Part model, mm, in its own coordinate system. A direction names the side the tool comes from. Coordinates: 2 decimals unless noted, no trailing zeros. Loops run counter-clockwise (first coordinate to the right, second up) from the corner with the lowest first, then second, coordinate; pieces in that order, holes last. Notation, with made-up numbers: M 55.25,64 L 62.25,64 A23 cw 62.25,84 Z; hole C -8,48 d10. An arc over 180 degrees is marked long. Use a Markdown table: item, result. Add a question column.
1) Band-saw the part on B-B (z = 39.65). List the corners of the cut face in (x, y), plus the area to 3 significant figures.
2) Tool access for faces 5 (the cylindrical face through (77.914, 10.793, 41.254)), 6 (the cylindrical face through (79.71, 37.57, 40.27)): list every direction of +Z, -Z, +X, -X, +Y, -Y with a clear straight run to the whole face (end or side of a thin tool).
3) Band-saw the part on C-C (x = 78.5). List the corners of the cut face in (y, z).
4) Pull direction X, two halves, no side cores. Call faces 1 (the cylindrical face through (80.873, 10.738, 40.268)), 2 (the cylindrical face through (79.419, 45.014, 40.014)), 3 (the flat face through (81, 10, 41.5)), 4 (the cylindrical face through (79.77, 36.52, 40.01)): released by +X, released by -X, zero draft, split by the parting line, or undercut.
5) Pin check, flat tips, straight feed: pin 1 Ø10 at (x, y) = (88.5, 14.5) entering from +Z; pin 2 Ø8 at (x, y) = (79.98, 30.02) entering from +Z. Stop position of each tip, or through.
6) Band-saw the part on A-A (y = 32). List the corners of the cut face in (x, z).
7) Band-saw the part on D-D (y = 37). List the corners of the cut face in (x, z), plus the area to 3 significant figures.
8) Wall check: probe 1 along X at (y, z) = (13, 39.1); probe 2 along Z at (x, y) = (92.5, 23.5); probe 3 along Y at (x, z) = (80.75, 39.5). Give the ranges that are in metal, low to high. Write a range as from..to.
from build123d import *

# Parameters (mm, degrees)
CYLINDER003001001005001001_R     = 3.5
CYLINDER003001001005001001_DEPTH = 2
CYLINDER003001001004002_R        = 1
CYLINDER003001001004002_DEPTH    = 5
CYLINDER003001001004001001_R     = 1
CYLINDER003001001004001001_DEPTH = 5
CYLINDER003001001005001_R        = 6.5
CYLINDER003001001005001_DEPTH    = 2
BOX002_W                         = 10
BOX002_H                         = 6
BOX002_DEPTH                     = 2
CYLINDER003001001004_R           = 2
CYLINDER003001001004_DEPTH       = 0.5
CYLINDER003001001004001_R        = 2
CYLINDER003001001004001_DEPTH    = 0.5
CYLINDER003001001005_R           = 15
CYLINDER003001001005_DEPTH       = 2
CUT002_ROLL_ANGLE                = 180
CUT002_PLACEMENT_ANGLE           = -90.233929


with BuildPart() as cylinder013:
    # Cylinder003001001005001001 → Cylinder003001001005001001 (new body)
    with BuildSketch(Plane(origin=(12, 6, 21), x_dir=(1, 0, 0), z_dir=(0, 0, 1))):
        Circle(CYLINDER003001001005001001_R)
    extrude(amount=CYLINDER003001001005001001_DEPTH)


with BuildPart() as cylinder014:
    # Cylinder003001001004002 → Cylinder003001001004002 (new body)
    with BuildSketch(Plane(origin=(-2.5, 6, 19.5), x_dir=(1, 0, 0), z_dir=(0, 0, 1))):
        Circle(CYLINDER003001001004002_R)
    extrude(amount=CYLINDER003001001004002_DEPTH)


with BuildPart() as cylinder015:
    # Cylinder003001001004001001 → Cylinder003001001004001001 (new body)
    with BuildSketch(Plane(origin=(25.5, 6, 19.5), x_dir=(1, 0, 0), z_dir=(0, 0, 1))):
        Circle(CYLINDER003001001004001001_R)
    extrude(amount=CYLINDER003001001004001001_DEPTH)


with BuildPart() as fusion009:
    # Cylinder003001001005001 → Cylinder003001001005001 (new body)
    with BuildSketch(Plane(origin=(6, 6, 21), x_dir=(1, 0, 0), z_dir=(0, 0, 1))):
        Circle(CYLINDER003001001005001_R)
    extrude(amount=CYLINDER003001001005001_DEPTH)

    # Fusion009: union Cylinder013, Cylinder014, Cylinder015
    add(cylinder013.part)
    add(cylinder014.part)
    add(cylinder015.part)


with BuildPart() as box002:
    # Box002 → Box002 (new body)
    with BuildSketch(Plane(origin=(18, 3, 21), x_dir=(1, 0, 0), z_dir=(0, 0, 1))):
        with Locations((5, 3)):
            Rectangle(BOX002_W, BOX002_H)
    extrude(amount=BOX002_DEPTH)


with BuildPart() as cylinder003001001004:
    # Cylinder003001001004 → Cylinder003001001004 (new body)
    with BuildSketch(Plane(origin=(-2.5, 6, 20.5), x_dir=(1, 0, 0), z_dir=(0, 0, 1))):
        Circle(CYLINDER003001001004_R)
    extrude(amount=CYLINDER003001001004_DEPTH)


with BuildPart() as cylinder010:
    # Cylinder003001001004001 → Cylinder003001001004001 (new body)
    with BuildSketch(Plane(origin=(25.5, 6, 20.5), x_dir=(1, 0, 0), z_dir=(0, 0, 1))):
        Circle(CYLINDER003001001004001_R)
    extrude(amount=CYLINDER003001001004001_DEPTH)


with BuildPart() as guide1:
    # Cylinder003001001005 → Cylinder003001001005 (new body)
    with BuildSketch(Plane(origin=(6, 6, 21), x_dir=(1, 0, 0), z_dir=(0, 0, 1))):
        Circle(CYLINDER003001001005_R)
    extrude(amount=CYLINDER003001001005_DEPTH)

    # Fusion008: union Box002, Cylinder003001001004, Cylinder010
    add(box002.part)
    add(cylinder003001001004.part)
    add(cylinder010.part)

    # Cut002: cut Fusion009
    add(fusion009.part, mode=Mode.SUBTRACT)


with BuildPart() as guide1_1:
    # Cut002 roll: moved
    add(guide1.part.rotate(Axis((0, 0, 0), (1, 0, 0)), CUT002_ROLL_ANGLE))


with BuildPart() as guide1_2:
    # Cut002 placement: moved
    add(guide1_1.part.moved(Location((86, 36, 62))).rotate(Axis((86, 36, 62), (0, 0, 1)), CUT002_PLACEMENT_ANGLE))


solid = guide1_2.part
Entries:
| question | item | result |
|---|---|---|
| 1 | outline | M 76.89,8.04 L 82.89,8.01 L 82.92,15.32 A15 ccw long 76.92,15.34 Z; hole M 76.49,24.54 A3.5 ccw long 83.42,24.51 A6.5 ccw long Z; hole C 79.9,10.52 d2; hole C 80.01,38.52 d2 |
| 1 | area | 592 mm2 |
| 2 | face 5 | +Z |
| 2 | face 6 | +Z, -Z |
| 3 | outline | M 8.03,39 L 20.84,39 L 20.84,41 L 11.96,41 L 11.96,41.5 L 9.09,41.5 L 9.09,41 L 8.03,41 Z; M 36.35,39 L 44.95,39 L 44.95,41 L 39.84,41 L 39.84,41.5 L 37.21,41.5 L 37.21,41 L 36.35,41 Z |
| 4 | face 1 | undercut |
| 4 | face 2 | split by the parting line |
| 4 | face 3 | zero draft |
| 4 | face 4 | undercut |
| 5 | pin 1 | z = 41 |
| 5 | pin 2 | through |
| 6 | outline | M 65.11,39 L 73.78,39 L 73.78,41 L 65.11,41 Z; M 86.17,39 L 94.84,39 L 94.84,41 L 86.17,41 Z |
| 7 | outline | M 66.7,39 L 93.25,39 L 93.25,41 L 81.3,41 L 81.3,41.5 L 78.72,41.5 L 78.72,41 L 66.7,41 Z |
| 7 | area | 54.4 mm2 |
| 8 | probe 1 | 76.91..82.91 |
| 8 | probe 2 | 39..41 |
| 8 | probe 3 | 8.02..10, 11.04..20.62, 36.48..37.85, 39.2..45 |
